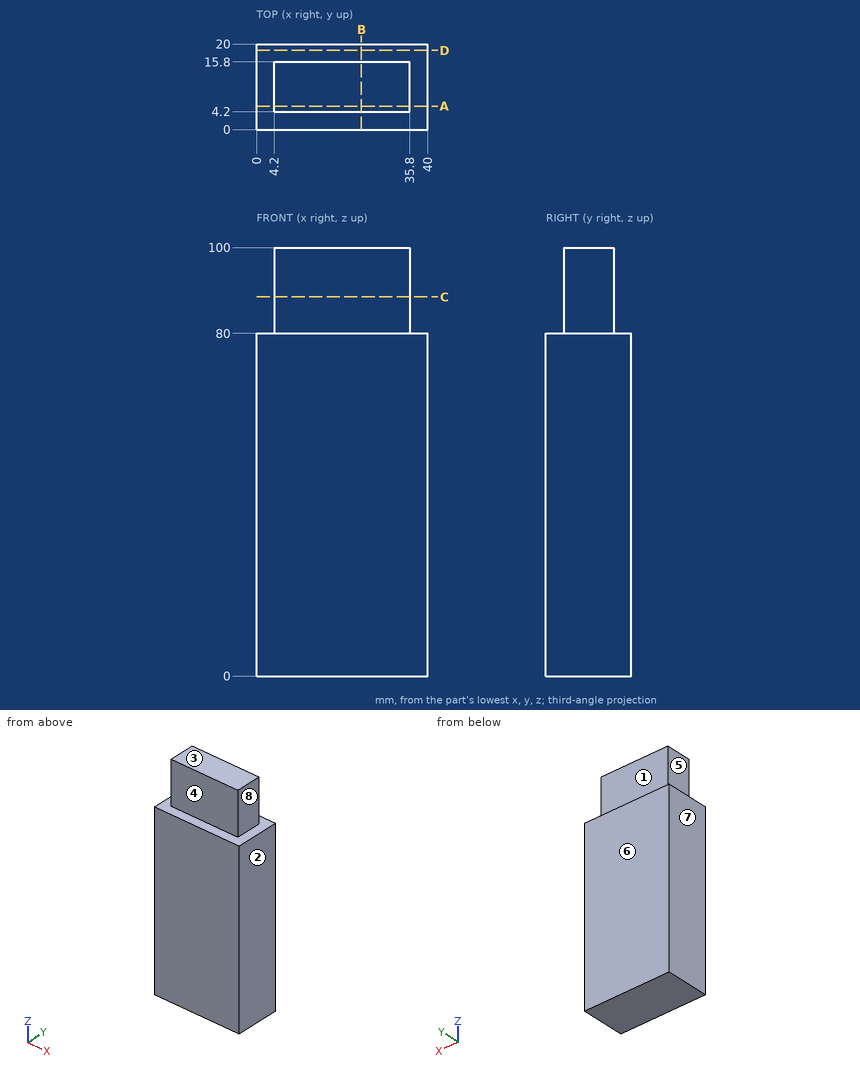
Print and shaded views of the part. All mm, measured from the part's lowest x, y and z. A direction names the side the tool comes from. Coordinates: 2 decimals unless noted, no trailing zeros. Loops run counter-clockwise (first coordinate to the right, second up) from the corner with the lowest first, then second, coordinate; pieces in that order, holes last. Notation, with made-up numbers: (74, 1) -> (93, 1) arc R16 ccw to (93, 13) -> close; hole circle Ø7 at (79, -27.75). An arc over 180 degrees is marked (long way). Use a Markdown table: item, result. Add a question column.
Item 1: Flat gauge pins, fed straight in: P1, Ø16, axis at x = 25, z = 90, coming from the -Y side; P2, Ø8, axis at x = 26, y = 11, coming from the -Z side; P3, Ø3.5, axis at y = 9, z = 86, coming from the -X side; P4, Ø3, axis at x = 17.5, y = 2.5, coming from the +Z side. Where does each tip first touch, or does it go through?
Item 2: Probe probe 1 along Z at (x, y) = (38, 4.75); probe 2 along Y at (x, z) = (7.5, 94). List the from-to ranges inside material, lowest first.
Item 3: Which spindle directions (+Z, -Z, +X, -X, +Y, -Y) get a long thin tool onto all of the face, cutting with end or side? Do the marked faces 1, 2, 3, 4 and 5. Say none if no direction does.
Item 4: Band-saw the part on B-B on x = 24.5. Write the cut outline in (y, z), plus the area to 3 significant figures.
Item 5: Pull direction X, two halves, no side cores. Call the marked faces 6, 7 and 8: +X half, -X half, draft (parallel to the pull), parting line (faces both ways), or undercut.
Item 6: Band-saw the part on A-A on y = 5.5. Write the cut outline in (x, z).
Item 7: Band-saw the part on C-C on z = 88.5. Write the cut outline in (x, y).
Item 8: Band-saw the part on D-D on y = 18.5. Write the cut outline in (x, z), plus the area to 3 significant figures.
Geometry says:
| question | item | result |
|---|---|---|
| 1 | P1 | y = 4.2 |
| 1 | P2 | z = 0 |
| 1 | P3 | x = 4.2 |
| 1 | P4 | z = 80 |
| 2 | probe 1 | 0 to 80 |
| 2 | probe 2 | 4.2 to 15.8 |
| 3 | face 1 | +Z, +X, -X, +Y |
| 3 | face 2 | +Z, -Z, +X, +Y, -Y |
| 3 | face 3 | +Z, +X, -X, +Y, -Y |
| 3 | face 4 | +Z, +X, -X, -Y |
| 3 | face 5 | +Z, -X, +Y, -Y |
| 4 | outline | (0, 0) -> (20, 0) -> (20, 80) -> (15.8, 80) -> (15.8, 100) -> (4.2, 100) -> (4.2, 80) -> (0, 80) -> close |
| 4 | area | 1,830 mm² |
| 5 | face 6 | draft |
| 5 | face 7 | -X half |
| 5 | face 8 | +X half |
| 6 | outline | (0, 0) -> (40, 0) -> (40, 80) -> (35.8, 80) -> (35.8, 100) -> (4.2, 100) -> (4.2, 80) -> (0, 80) -> close |
| 7 | outline | (4.2, 4.2) -> (35.8, 4.2) -> (35.8, 15.8) -> (4.2, 15.8) -> close |
| 8 | outline | (0, 0) -> (40, 0) -> (40, 80) -> (0, 80) -> close |
| 8 | area | 3,200 mm² |
